Source: CAD feature listing. Evaluate the final solid. Frame: model axes, mm. A direction names the side the tool comes from. Round coordinates to 2 decimals unless told otherwise and drop trailing zeros. Order: outer loops, then holes, each group sorted by start corner. A loop starts at its lowest first (then second) coordinate and runs counter-clockwise, first axis right, second up. Notation, with made-up numbers: (-32.5, 55.5) -> (9.5, 55.5) arc R21 cw to (9.5, 83.5) -> close; hole circle Ø1 at (33, -27.5). An arc over 180 degrees is marked (long way). Answer as CSV lines item,"result". Start each with the question number.
(1) Section query A-A (x = -20). Output: boundary loops of the cut face in (y, z), plus the area to 3 significant figures.
(2) Section query B-B (z = -2.25). Output: boundary loops of the cut face in (x, y), plus the area to 3 significant figures.
(3) Section query C-C (y = 7). Output: boundary loops of the cut face in (x, z), plus the area to 3 significant figures.
(4) Contact query for flat-ended pins moving along their axis: P1, Ø3, axis at x = -18.5, y = -9, coming from the -Z side; P2, Ø4, axis at y = -3, z = 2.5, coming from the +X side; P3, Ø5, axis at y = 113, z = 2, coming from the +X side; P4, Ø6, axis at y = 26.5, z = 2.5, coming from the -X side. Output: stop coordinate, or through.
(5) Set-up query: faces 1 (the cylindrical face through (22.4, 7.1, 2.6)), 2 (the flat face through (-6.681, 115, 0)), 3 (the cylindrical face through (22.4, 7.1, -2.6)), 4 (the flat face through (4.819, 115, 0)), 5 (the cylindrical face through (-22.116, 0.973, 0.002)). Return all of +Z, -Z, +X, -X, +Y, -Y with unobstructed straight access to the full face (end or side cutting, diameter ignored); none if empty.
(6) Line query: line 1 along Y through (x, z) = (1, 2); line 2 along Y through (x, z) = (4, -0.5); line 3 along X through (y, z) = (-27, 4). Output: solid intervals per line, ascending. Write a range as from..to.
(7) Pull-direction query (X, two-part tool) for faces 6 (the flat face through (16, 16, -0.17)), 7 (the flat face through (0, 27, -5)), 8 (the cylindrical face through (-0.76, -34.49, 0.07)), 9 (the flat face through (-20.396, 55.39, 0.07)); classes: +X half, -X half, draft (parallel to the pull), parting line (faces both ways), or undercut.
(8) Section query D-D (x = 25.5). Output: boundary loops of the cut face in (y, z).
```python
from build123d import *

# Parameters (mm, degrees)
BOSS_EXTRUDE1_DEPTH     = 5
CUT_EXTRUDE1_START      = 5
SKETCH2_R               = 23.5
CUT_EXTRUDE1_DEPTH      = 4.83
CUT_EXTRUDE2_START      = -5
SKETCH2_2_R             = 23.5
CUT_EXTRUDE2_DEPTH      = 4.83
SKETCH3_R               = 22.1375
CUT_EXTRUDE3_DEPTH      = 6
CUT_EXTRUDE3_DEPTH_BACK = 6


with BuildPart() as part:
    # Sketch1 → Boss-Extrude1 (new body, symmetric)
    with BuildSketch(Plane.XY):
        with BuildLine():
            Line((4.819095737, 120.75), (-6.680904263, 120.75))
            Line((-6.680904263, 120.75), (-6.680904263, 109.25))
            Line((-6.680904263, 109.25), (-34.5, 0))
            ThreePointArc((-34.5, 0), (0, -34.5), (34.5, 0))
            Line((34.5, 0), (4.819095737, 109.25))
            Line((4.819095737, 109.25), (4.819095737, 120.75))
        make_face()
    extrude(amount=BOSS_EXTRUDE1_DEPTH, both=True)

    # Sketch2 → Cut-Extrude1 (cut)
    with BuildSketch(Plane.XY.offset(CUT_EXTRUDE1_START)):
        Circle(SKETCH2_R)
    extrude(amount=-CUT_EXTRUDE1_DEPTH, mode=Mode.SUBTRACT)

    # Sketch2<2> → Cut-Extrude2 (cut)
    with BuildSketch(Plane.XY.offset(CUT_EXTRUDE2_START)):
        Circle(SKETCH2_2_R)
    extrude(amount=CUT_EXTRUDE2_DEPTH, mode=Mode.SUBTRACT)

    # Sketch3 → Cut-Extrude3 (cut, two sides)
    with BuildSketch(Plane.XY) as cut_extrude3_sk:
        Circle(SKETCH3_R)
    extrude(amount=CUT_EXTRUDE3_DEPTH, mode=Mode.SUBTRACT)
    extrude(cut_extrude3_sk.sketch, amount=-CUT_EXTRUDE3_DEPTH_BACK, mode=Mode.SUBTRACT)


solid = part.part
```
Answer block:
1,outline,"(-28.11, -5) -> (-12.34, -5) -> (-12.34, -0.17) -> (-9.49, -0.17) -> (-9.49, 0.17) -> (-12.34, 0.17) -> (-12.34, 5) -> (-28.11, 5) -> close; (9.49, -0.17) -> (12.34, -0.17) -> (12.34, -5) -> (56.94, -5) -> (56.94, 5) -> (12.34, 5) -> (12.34, 0.17) -> (9.49, 0.17) -> close"
1,area,"606 mm2"
2,outline,"(-34.5, 0) arc R34.5 ccw to (34.5, 0) -> (4.82, 109.25) -> (4.82, 120.75) -> (-6.68, 120.75) -> (-6.68, 109.25) -> close; hole circle Ø47 at (0, 0)"
2,area,"4,660 mm2"
3,outline,"(-32.72, -5) -> (-22.43, -5) -> (-22.43, -0.17) -> (-21, -0.17) -> (-21, 0.17) -> (-22.43, 0.17) -> (-22.43, 5) -> (-32.72, 5) -> close; (21, -0.17) -> (22.43, -0.17) -> (22.43, -5) -> (32.6, -5) -> (32.6, 5) -> (22.43, 5) -> (22.43, 0.17) -> (21, 0.17) -> close"
3,area,"205 mm2"
4,P1,"through"
4,P2,"x = 34.49"
4,P3,"x = 4.82"
4,P4,"x = -28.52"
5,face 1,"+Z"
5,face 2,"+Z, -Z, -X, +Y"
5,face 3,"-Z"
5,face 4,"+Z, -Z, +X, +Y"
5,face 5,"+Z, -Z"
6,line 1,"-34.49..-23.48, 23.48..120.75"
6,line 2,"-34.27..-23.16, 23.16..120.75"
6,line 3,"-21.48..21.48"
7,face 6,"undercut"
7,face 7,"draft"
7,face 8,"parting line"
7,face 9,"-X half"
8,outline,"(-23.24, -5) -> (33.13, -5) -> (33.13, 5) -> (-23.24, 5) -> close"
